Here's the drawing with two shaded views (mm, measured from the low corner). I have some questions. A direction names the side the tool comes from. Round coordinates to 2 decimals unless told otherwise and drop trailing zeros. Loops run counter-clockwise (first coordinate to the right, second up) from the corner with the lowest first, then second, coordinate; pieces in that order, holes last.
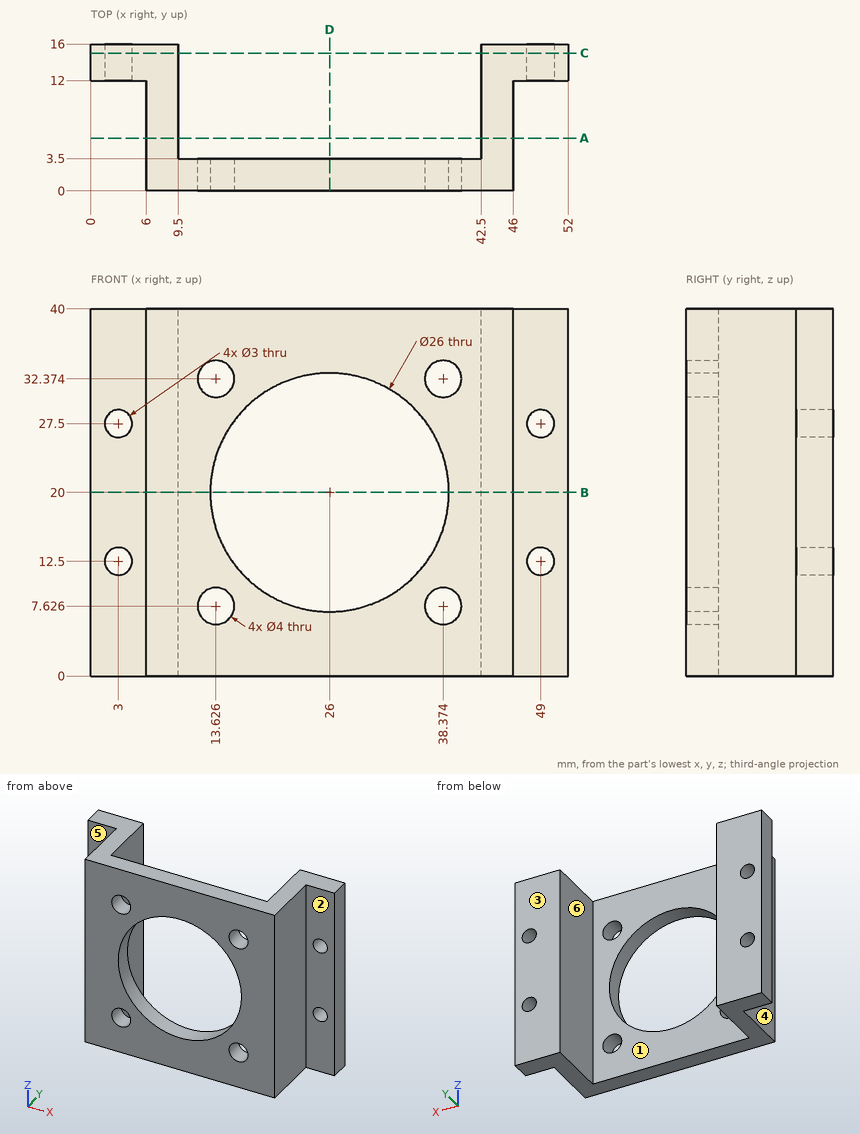
(1) If we section it at C-C, the plane y = 15: List the corners of the cut face in (x, z) for me.
Worked answers:
outline: (0, 0) - (9.5, 0) - (9.5, 40) - (0, 40) - close; (42.5, 0) - (52, 0) - (52, 40) - (42.5, 40) - close; hole circle Ø3 at (3, 12.5); hole circle Ø3 at (3, 27.5); hole circle Ø3 at (49, 12.5); hole circle Ø3 at (49, 27.5)
(2) If we section it at A-A, the plane y = 5.75: List the corners of the cut face in (x, z) for me.
Worked answers:
outline: (6, 0) - (9.5, 0) - (9.5, 40) - (6, 40) - close; (42.5, 0) - (46, 0) - (46, 40) - (42.5, 40) - close
(3) If we section it at B-B, the plane z = 20: List the corners of the cut face in (x, y) for me.
Worked answers:
outline: (0, 12) - (6, 12) - (6, 0) - (13, 0) - (13, 3.5) - (9.5, 3.5) - (9.5, 16) - (0, 16) - close; (39, 0) - (46, 0) - (46, 12) - (52, 12) - (52, 16) - (42.5, 16) - (42.5, 3.5) - (39, 3.5) - close
(4) For the marked faces 1, 2 and 3, which set-ups out of +Z, -Z, +X, -X, +Y, -Y let a thin tool reach every point of the face, with its end or its side?
Worked answers:
face 1: +Z, -Z, +Y
face 2: +Z, -Z, +X, -Y
face 3: +Z, -Z, +X, -X, +Y
(5) Will these pins go through, and if not, where does the flat tip stop? P1, Ø3.5, axis at y = 3.5, z = 23.5, coming from the +X side; P2, Ø4.5, axis at x = 13.63, z = 7.63, coming from the +Y side; P3, Ø3.5, axis at x = 38.37, z = 32.37, coming from the -Y side; P4, Ø3.5, axis at x = 3, z = 27.5, coming from the -Y side.
Worked answers:
P1: stops at x = 46
P2: stops at y = 3.5
P3: passes through
P4: stops at y = 12
(6) If we mould it in two halves opening along X, with no side actions, what happens to the marked faces 4, 5 and 6? For each: released by +X, released by -X, zero draft, split by the parting line, or undercut.
Worked answers:
face 4: released by -X
face 5: zero draft
face 6: undercut
(7) If we section it at D-D, the plane x = 26: List the corners of the cut face in (y, z) for me.
Worked answers:
outline: (0, 0) - (3.5, 0) - (3.5, 7) - (0, 7) - close; (0, 33) - (3.5, 33) - (3.5, 40) - (0, 40) - close
(8) If I drill on line 1 (Z direction, x = 3, y = 13.55); line 2 (X direction, y = 7, z = 6.5); line 3 (X direction, y = 14.5, z = 6), over which ranges is the centre line in solid material (lowest first)?
Worked answers:
line 1: z = 0 to 11, 14 to 26, 29 to 40
line 2: x = 6 to 9.5, 42.5 to 46
line 3: x = 0 to 9.5, 42.5 to 52
